Work out the finished part from the listing and answer in its coordinate system (mm). Round coordinates to 2 decimals unless told otherwise and drop trailing zeros. Write each loop counter-clockwise with the first axis right and the second up, starting at its lowest first coordinate (ties: lowest second). Pieces come first, ordered by that corner, then holes. Notation, with made-up numbers: (-0.75, 2.5) - (56.25, 2.5) arc R20 ccw to (56.25, 32.5) - close; hole circle Ø5 at (60.5, -15.75). An arc over 180 degrees is marked (long way). Answer as a JSON object with one key per item and string values.
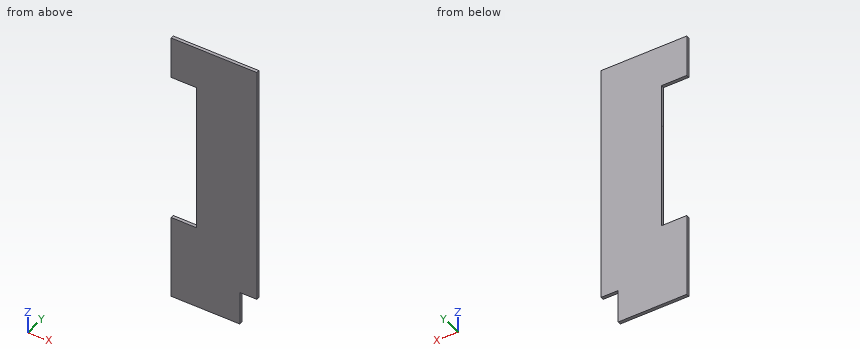
Autodesk Inventor part; units mm, degrees
ref_plane "YZ Plane" through (0, 0, 0) normal (1, 0, 0) x (0, 1, 0)
ref_plane "XZ Plane" through (0, 0, 0) normal (0, 1, 0) x (-1, 0, 0)
ref_plane "XY Plane" through (0, 0, 0) normal (0, 0, 1) x (1, 0, 0)
sketch "Sketch1" plane through (0, 0, 0) normal (0, 1, 0) x (-1, 0, 0)
  line L0 (542.2576, 149.421) -> (414.2963, 149.421)
  line L1 (414.2963, 149.421) -> (414.2963, -266.7891)
  line L2 (414.2963, -266.7891) -> (542.2576, -266.7891)
  line L3 (542.2576, -266.7891) -> (542.2576, 149.421)
  point P0 (0, 0)
extrude "Extrusion1" add sketch "Sketch1" along normal blind 4.7498
sketch "Sketch2" plane through (0, 0, 0) normal (0, -1, 0) x (1, 0, 0)
  point P0 (0, 0)
sketch "Sketch3" plane through (0, 0, 0) normal (0, -1, 0) x (1, 0, 0)
  line L0 (-542.2576, 149.421) -> (-414.2963, 149.421)
  line L1 (-542.2576, 149.421) -> (-542.2576, 22.421)
  line L2 (-542.2576, -266.7891) -> (-542.2576, 149.421)
  line L3 (-414.2963, -266.7891) -> (-542.2576, -266.7891)
  line L4 (-542.2576, -266.7891) -> (-542.2576, -139.7891)
  line L5 (-542.2576, -139.7891) -> (-504.1576, -139.7891)
  line L6 (-504.1576, -139.7891) -> (-504.1576, 22.421)
  line L7 (-504.1576, 22.421) -> (-542.2576, 22.421)
  line L8 (-504.1576, -139.7891) -> (-542.2576, -139.7891)
  line L9 (-542.2576, -139.7891) -> (-542.2576, 22.421)
  line L10 (-542.2576, 22.421) -> (-504.1576, 22.421)
  line L11 (-504.1576, 22.421) -> (-504.1576, -139.7891)
  point P0 (0, 0)
  dimension "d2" = 127
  dimension "d3" = 127
  dimension "d4" = 38.1
extrude "Extrusion2" cut sketch "Sketch3" against normal blind 65.0875
sketch "Sketch4" plane through (0, 0, 0) normal (0, -1, 0) x (1, 0, 0)
  point P0 (0, 0)
sketch "Sketch5" plane through (0, 0, 0) normal (0, -1, 0) x (1, 0, 0)
  line L0 (-542.2576, 22.421) -> (-542.2576, 85.921)
  line L1 (-542.2576, 22.421) -> (-542.2576, 149.421)
  line L2 (-510.2194, 85.921) -> (-510.2194, 22.421)
  line L3 (-542.2576, 22.421) -> (-504.1576, 22.421)
  line L4 (-542.2576, 85.921) -> (-510.2194, 85.921)
  point P0 (0, 0)
sketch "Sketch6" plane through (0, 0, 0) normal (0, -1, 0) x (1, 0, 0)
  point P0 (0, 0)
extrude "Extrusion3" cut sketch "Sketch5" against normal blind 123.825
sketch "Sketch7" plane through (0, 4.7498, 0) normal (0, 1, 0) x (1, 0, 0)
  line L0 (-414.2963, -149.421) -> (-414.2963, 266.7891)
  line L1 (-414.2963, 266.7891) -> (-433.3463, 266.7891)
  line L2 (-414.2963, 266.7891) -> (-542.2576, 266.7891)
  line L3 (-433.3463, 266.7891) -> (-433.3463, 215.9891)
  line L4 (-433.3463, 215.9891) -> (-414.2963, 215.9891)
  point P0 (0, 0)
  dimension "d9" = 19.05
  dimension "d11" = 50.8
extrude "Extrusion4" cut sketch "Sketch7" against normal blind 42.8625
sketch "Sketch8" plane through (0, 4.7498, 0) normal (0, 1, 0) x (1, 0, 0)
  line L0 (-510.2194, -22.421) -> (-504.1207, -22.421)
  line L1 (-504.1207, -22.421) -> (-504.1207, -85.7832)
  line L2 (-510.2194, -85.921) -> (-510.2194, -22.421)
  line L3 (-510.2194, -85.7832) -> (-510.2194, -22.421)
  line L4 (-542.2576, -85.921) -> (-510.2194, -85.921)
  line L5 (-510.2194, -85.7832) -> (-510.2194, -85.921)
  line L6 (-510.2194, -85.921) -> (-504.1207, -85.921)
  line L7 (-504.1207, -85.921) -> (-504.1207, -85.7832)
  point P0 (0, 0)
extrude "Extrusion5" cut sketch "Sketch8" against normal blind 28.575
sketch "Sketch9" plane through (0, 4.7498, 0) normal (0, 1, 0) x (1, 0, 0)
  point P0 (0, 0)
sketch "Sketch10" plane through (0, 4.7498, 0) normal (0, 1, 0) x (1, 0, 0)
  line L0 (-414.2963, 215.9891) -> (-433.3463, 215.9891)
  line L1 (-433.3463, 215.9891) -> (-439.6963, 215.9891)
  line L2 (-439.6963, 215.9891) -> (-439.6963, 266.7891)
  line L3 (-433.3463, 266.7891) -> (-542.2576, 266.7891)
  line L4 (-433.3463, 266.7891) -> (-433.3463, 215.9891)
  line L5 (-433.3463, 266.7891) -> (-433.3463, 215.9891)
  point P0 (0, 0)
  dimension "d16" = 6.35
extrude "Extrusion6" cut sketch "Sketch10" against normal blind 36.5125
properties part number "Lexan" material "Acetal Resin, White(1)"
Item 1: A cutting plane is placed at D-D (z = 31). Write down the section's boundary in (x, y).
Results found:
{"outline": "(-504.12, 0) - (-414.3, 0) - (-414.3, 4.75) - (-504.12, 4.75) - close"}
Item 2: A cutting plane is placed at A-A (x = -521). Write down the section's boundary in (y, z).
Results found:
{"outline": "(0, -266.79) - (4.75, -266.79) - (4.75, -139.79) - (0, -139.79) - close; (0, 85.92) - (4.75, 85.92) - (4.75, 149.42) - (0, 149.42) - close"}
Item 3: Consider line 1 along Z through (x, y) = (-524.5, 1.5); line 2 along X through (y, z) = (2.95, -52); line 3 along Z through (x, y) = (-439.5, 0.2). Determine where each line is inside the solid, lowest interval first.
Results found:
{"line 1": "-266.79 to -139.79, 85.92 to 149.42", "line 2": "-504.16 to -414.3", "line 3": "-215.99 to 149.42"}
Item 4: A cutting plane is placed at C-C (z = -13). Write down the section's boundary in (x, y).
Results found:
{"outline": "(-504.16, 0) - (-414.3, 0) - (-414.3, 4.75) - (-504.16, 4.75) - close"}
Item 5: This flat-tipped pin is pushed along its axis until it touches: P1, Ø1, axis at x = -469.5, z = -64.5, coming from the -Y side. Where does it stop, or does it pass through?
Results found:
{"P1": "y = 0"}
